Autodesk Inventor part; units mm, degrees
ref_plane "YZ Plane" through (0, 0, 0) normal (1, 0, 0) x (0, 1, 0)
ref_plane "XZ Plane" through (0, 0, 0) normal (0, 1, 0) x (-1, 0, 0)
ref_plane "XY Plane" through (0, 0, 0) normal (0, 0, 1) x (1, 0, 0)
sketch "Boceto1" plane through (0, 0, 0) normal (0, 1, 0) x (-1, 0, 0)
  line L0 (-3.175, 6) -> (3.175, 6)
  line L1 (3.175, 6) -> (3.175, -6)
  line L2 (3.175, -6) -> (-3.175, -6)
  line L3 (-3.175, -6) -> (-3.175, 6)
  line L4 (-3.175, 6) -> (3.175, -6) construction
  line L5 (3.175, 6) -> (-3.175, -6) construction
  line L6 (8.175, 6) -> (-8.175, 6)
  line L7 (-8.175, 6) -> (-8.175, -6)
  line L8 (-8.175, -6) -> (8.175, -6)
  line L9 (8.175, -6) -> (8.175, 6)
  circle A0 centre (5.7194, 3) radius 1.65
  circle A1 centre (5.7194, -3) radius 1.65
  circle A2 centre (-5.6782, 3) radius 1.65
  circle A3 centre (-5.6782, -3) radius 1.65
  point P0 (0, 0)
  dimension "d0" = 6.35
  dimension "d1" = 12
  dimension "d2" = 5
  dimension "d3" = 5
  dimension "d4" = 3.3
  dimension "d5" = 3
  dimension "d6" = 3
extrude "Extrusión1" add sketch "Boceto1" along normal blind 3
sketch "Boceto2" plane through (0, 3, 0) normal (0, 1, 0) x (1, 0, 0)
  line L0 (8.175, 6) -> (-8.175, 6)
  line L1 (3.175, -6) -> (-3.175, -6)
  line L2 (-3.175, -6) -> (-3.175, 6)
  line L3 (-3.175, 6) -> (3.175, 6)
  line L4 (3.175, 6) -> (3.175, -6)
  line L5 (3.175, -6) -> (-3.175, 6) construction
  line L6 (-3.175, -6) -> (3.175, 6) construction
  point P0 (0, 0)
  dimension "d9" = 6.35
extrude "Extrusión2" cut sketch "Boceto2" against normal blind 1
fillet "Empalme1" radius 2 4 edges at (-8.175, 1.5, 6) (8.175, 1.5, 6) (8.175, 1.5, -6) (-8.175, 1.5, -6)
properties part number "lockbelt"
Verification items for the finished model (mm, model axes). A direction names the side the tool comes from. Coordinates: 2 decimals unless noted, no trailing zeros. Loops run counter-clockwise (first coordinate to the right, second up) from the corner with the lowest first, then second, coordinate; pieces in that order, holes last. Notation, with made-up numbers: (75, 68.25) - (122, 68.25) arc R7 cw to (122, 79.25) - close; hole circle Ø2 at (1.25, 2.5). An arc over 180 degrees is marked (long way). Answer as a JSON object with one key per item and string values.
(1) Cross-section at A-A, the plane y = 2.8. Record the boundary of the cut face in (x, z) (3 decimals), then the cut area to 3 significant figures.
Response:
{"outline": "(-8.175, -4) arc R2 ccw to (-6.175, -6) - (-3.175, -6) - (-3.175, 6) - (-6.175, 6) arc R2 ccw to (-8.175, 4) - close; (3.175, -6) - (6.175, -6) arc R2 ccw to (8.175, -4) - (8.175, 4) arc R2 ccw to (6.175, 6) - (3.175, 6) - close; hole circle Ø3.3 at (-5.719, -3); hole circle Ø3.3 at (-5.719, 3); hole circle Ø3.3 at (5.678, -3); hole circle Ø3.3 at (5.678, 3)", "area": "82.4 mm²"}
(2) Mould release check, pull along X, two halves, no side actions. Record for faces 1 (the cylindrical face through (-7.574, 1.521, -5.43)), 2 (the flat face through (0, 2, 0)), 3 (the flat face through (0, 1, 6)): pulls with the +X half, pulls with the -X half, needs draft (parallel to the pull), parting line crosses it, or undercut.
Response:
{"face 1": "pulls with the -X half", "face 2": "undercut", "face 3": "needs draft"}
(3) Cross-section at B-B, the plane y = 1.5. Record the boundary of the cut face in (x, z) (3 decimals).
Response:
{"outline": "(-8.175, -4) arc R2 ccw to (-6.175, -6) - (6.175, -6) arc R2 ccw to (8.175, -4) - (8.175, 4) arc R2 ccw to (6.175, 6) - (-6.175, 6) arc R2 ccw to (-8.175, 4) - close; hole circle Ø3.3 at (-5.719, -3); hole circle Ø3.3 at (-5.719, 3); hole circle Ø3.3 at (5.678, -3); hole circle Ø3.3 at (5.678, 3)"}
(4) Cross-section at D-D, the plane x = 5.75. Record the boundary of the cut face in (y, z).
Response:
{"outline": "(0, -6) - (3, -6) - (3, -4.65) - (0, -4.65) - close; (0, -1.35) - (3, -1.35) - (3, 1.35) - (0, 1.35) - close; (0, 4.65) - (3, 4.65) - (3, 6) - (0, 6) - close"}
(5) Access from +Z, -Z, +X, -X, +Y, -Y to the whole of each face (thin tool, end or side, straight path). Record for faces 4 (the cylindrical face through (7.327, 1.479, 2.927)), 5 (the flat face through (-3.175, 2.5, 0.1)).
Response:
{"face 4": "+Y, -Y", "face 5": "+Z, -Z, +Y"}
(6) Go/stop test with flat-tipped pins: pin 1 Ø1.9 at (x, z) = (1, 0) entering from +Y; pin 2 Ø3 at (x, z) = (5.68, 3) entering from +Y. Record where each tip stops, or that it passes through.
Response:
{"pin 1": "stops at y = 2", "pin 2": "passes through"}
(7) Cross-section at C-C, the plane z = -3. Record the boundary of the cut face in (x, y) (3 decimals).
Response:
{"outline": "(-8.175, 0) - (-7.369, 0) - (-7.369, 3) - (-8.175, 3) - close; (-4.069, 0) - (4.028, 0) - (4.028, 3) - (3.175, 3) - (3.175, 2) - (-3.175, 2) - (-3.175, 3) - (-4.069, 3) - close; (7.328, 0) - (8.175, 0) - (8.175, 3) - (7.328, 3) - close"}
(8) Scan lines: line 1 along X through (y, z) = (1.8, -2.5) (3 decimals); line 2 along X through (y, z) = (0.55, 3.75) (1 decimal); line 3 along Z through (x, y) = (6.75, 0.8). Record each from-to range of solid material in increasing order.
Response:
{"line 1": "x = -8.175 to -7.292, -4.147 to 4.106, 7.251 to 8.175", "line 2": "x = -8.2 to -7.2, -4.2 to 4.2, 7.1 to 8.2", "line 3": "z = -5.92 to -4.25, -1.75 to 1.75, 4.25 to 5.92"}
